Could you check a few things on this model? Use its own coordinates, in mm. Coordinates: 2 decimals unless noted, no trailing zeros. Loops run counter-clockwise (first coordinate to the right, second up) from the corner with the lowest first, then second, coordinate; pieces in that order, holes last. Notation, with made-up numbers: M 41,-23 L 49,-23 A23 ccw 49,4 Z; hole C -10,75 d9. An arc over 180 degrees is marked long. Return JSON: item names as keys, results as strings. Group by question number.
from build123d import *

# Parameters (mm, degrees)
SKETCH_1_W               = 20
SKETCH_1_H               = 20
EXTRUDE_1_DEPTH          = 275.47
CUT_EXTRUDE_1_DEPTH      = 263.92
CUT_EXTRUDE_2_DEPTH      = 277.918256711
CUT_EXTRUDE_2_DEPTH_BACK = 277.918256711
SKETCH_3_R               = 2
SKETCH_3_R_2             = 2.15
SKETCH_4_R               = 2.1
CUT_EXTRUDE_3_DEPTH      = 60


with BuildPart() as part:
    # 草图1 → 凸台-拉伸1 (new body)
    with BuildSketch(Plane.XY):
        with Locations((10, 10)):
            Rectangle(SKETCH_1_W, SKETCH_1_H)
    extrude(amount=EXTRUDE_1_DEPTH)

    # 草图2 → 切除-拉伸1 (cut)
    with BuildSketch(Plane(origin=(0, 20, 0), x_dir=(1, 0, 0), z_dir=(0, 1, 0))):
        Polygon((0, -275.47), (20, -240.828983849), (20, -275.47), align=None)
        Polygon((20, 0), (0, -11.547005384), (0, 0), align=None)
    extrude(amount=-CUT_EXTRUDE_1_DEPTH, mode=Mode.SUBTRACT)

    # 草图3 → 切除-拉伸2 (cut, two sides: drawn at the far end of the back side and taken through both)
    with BuildSketch(Plane.XZ.offset(-CUT_EXTRUDE_2_DEPTH_BACK)):
        with Locations(Location((10, 239.74, 0), (0, 0, 270))):
            Circle(SKETCH_3_R)
        with Locations(Location((10, 224.74, 0), (0, 0, 270))):
            Circle(SKETCH_3_R)
        with Locations(Location((10, 194.74, 0), (0, 0, 270))):
            Circle(SKETCH_3_R)
        with Locations(Location((10, 174.74, 0), (0, 0, 270))):
            Circle(SKETCH_3_R_2)
    extrude(amount=CUT_EXTRUDE_2_DEPTH + CUT_EXTRUDE_2_DEPTH_BACK, mode=Mode.SUBTRACT)

    # 草图4 → 切除-拉伸3 (cut)
    with BuildSketch(Plane.XZ):
        with Locations(Location((10, 21.547005384, 0), (0, 0, 270))):
            Circle(SKETCH_4_R)
        with Locations(Location((10, 41.547005384, 0), (0, 0, 270))):
            Circle(SKETCH_4_R)
    extrude(amount=-CUT_EXTRUDE_3_DEPTH, mode=Mode.SUBTRACT)


solid = part.part
(1) Imagine slicing it at C-C, the plane z = 248. Write out the boundary of the cut face in (x, y), then the cut area to 3 significant figures.
(2) Imagine slicing it at B-B, the plane x = 17.75. Write out the boundary of the cut face in (y, z), then the cut area to 3 significant figures.
(3) We'd pull the mould along X, two halves only. Please class faces 1 (the face through (10.14, 10.14, 5.693)), 2 (the face through (11.77, 9.86, 40.42)), 3 (the face through (10, 20, 136)), 4 (the face through (9.177, 10.14, 172.754)): +X half, -X half, draft (parallel to the pull), parting line (faces both ways), or undercut.
(4) Will this pin go through, and if not, where does the flat tip stop? P1, Ø6, axis at x = 12, y = 6.5, coming from the +Z side.
(5) Imagine slicing it at A-A, the plane y = 10.5. Write out the boundary of the cut face in (x, z).
(6) If I drill on L1, parallel to X at y = 11, z = 224.74; L2, parallel to Z at x = 1, y = 2; L3, parallel to Z at x = 6.25, y = 16.25, over which ranges is the centre line in solid material (lowest first)? Write a range as [from, to].
Checks:
{
 "1": {"outline": "M 0,0 L 15.86,0 L 15.86,20 L 0,20 Z", "area": "317 mm²"},
 "2": {"outline": "M 0,1.3 L 20,1.3 L 20,244.73 L 0,244.73 Z", "area": "4,870 mm²"},
 "3": {"face 1": "-X half", "face 2": "undercut", "face 3": "draft", "face 4": "undercut"},
 "4": {"P1": "z = 259.88"},
 "5": {"outline": "M 0,11.55 L 20,0 L 20,240.83 L 0,275.47 Z; hole C 10,174.74 d4.3; hole C 10,21.55 d4.2; hole C 10,41.55 d4.2; hole C 10,194.74 d4; hole C 10,224.74 d4; hole C 10,239.74 d4"},
 "6": {"L1": "[0, 8], [12, 20]", "L2": "[10.97, 273.74]", "L3": "[7.94, 264.64]"}
}
